```python
from build123d import *

# Parameters (mm, degrees)
F0_R     = 31.5
F0_R_2   = 26.5
F1_DEPTH = 25
F2_R     = 37
F2_R_2   = 31.5
F2_R_3   = 26.5
F3_DEPTH = 5
F4_R     = 1
F5_R     = 1
F6_R     = 5


with BuildPart() as f1:
    # F0 (on Top) → F1 (new body)
    with BuildSketch(Plane.XY):
        Circle(F0_R)
        Circle(F0_R_2, mode=Mode.SUBTRACT)
    extrude(amount=F1_DEPTH)

    # F2 (on face) → F3 (join)
    with BuildSketch(Plane.XY.offset(25)):
        Circle(F2_R)
        Circle(F2_R_2, mode=Mode.SUBTRACT)
        Circle(F2_R_2)
        Circle(F2_R_3, mode=Mode.SUBTRACT)
        Circle(F2_R_3)
    extrude(amount=F3_DEPTH)

    # F4
    f4_edges = [f1.edges().sort_by_distance(p)[0] for p in [
        (-37, 0, 30),
    ]]
    fillet(f4_edges, radius=F4_R)

    # F5
    f5_edges = [f1.edges().sort_by_distance(p)[0] for p in [
        (-31.5, 0, 0),
    ]]
    fillet(f5_edges, radius=F5_R)

    # F6
    f6_edges = [f1.edges().sort_by_distance(p)[0] for p in [
        (-26.5, 0, 25),
    ]]
    fillet(f6_edges, radius=F6_R)


solid = f1.part
```
Geometry check sheet. Reference: the model listing, model coordinates, mm. A direction names the side the tool comes from. Round coordinates to 2 decimals unless told otherwise and drop trailing zeros. Order: outer loops, then holes, each group sorted by start corner. A loop starts at its lowest first (then second) coordinate and runs counter-clockwise, first axis right, second up. Notation, with made-up numbers: M -12,44.25 L 5,44.25 A25 cw 5,79.25 Z; hole C 56,-24 d1. An arc over 180 degrees is marked long. Answer as CSV lines item,"result".
1) Tool access check on faces 1 (the face through (-8.02, -36.12, 26.97)), 2 (the face through (27, 17, 25)). Record the directions out of +Z, -Z, +X, -X, +Y, -Y that give a thin tool (end or side, any length) a straight path to the whole face; none if there is none.
Entries:
face 1,"+Z, -Z"
face 2,"-Z"
2) Sectioned sample at A-A on x = 0. Record the cut outline in (y, z).
Entries:
outline,"M -37,25 L -31.5,25 L -31.5,1 A1 ccw -30.5,0 L -26.5,0 L -26.5,20 A5 cw -21.5,25 L 21.5,25 A5 cw 26.5,20 L 26.5,0 L 30.5,0 A1 ccw 31.5,1 L 31.5,25 L 37,25 L 37,29 A1 ccw 36,30 L -36,30 A1 ccw -37,29 Z"
3) Sectioned sample at D-D on z = 26. Record the cut outline in (x, y), and give its area (3 significant figures).
Entries:
outline,"C 0,0 d74"
area,"4,300 mm2"
4) Mould release check, pull along Y, two halves, no side actions. Record for faces 3 (the face through (14.246, 22.345, 9.86)), 4 (the face through (-4.101, 31.232, 12.832)), 5 (the face through (-23, 14, 0)): +Y half, -Y half, draft (parallel to the pull), parting line (faces both ways), or undercut.
Entries:
face 3,"undercut"
face 4,"parting line"
face 5,"draft"
5) Sectioned sample at C-C on z = 10.5. Record the cut outline in (x, y), and give its area (3 significant figures).
Entries:
outline,"C 0,0 d63; hole C 0,0 d53"
area,"911 mm2"
6) Thickness scan on probe 1 along Y at (x, z) = (0, 10.25); probe 2 along X at (y, z) = (4, 19.5) (3 decimals); probe 3 along Z at (x, y) = (14.5, 1.5). Record the ranges inside material, lowest first. Write a range as [from, to].
Entries:
probe 1,"[-31.5, -26.5], [26.5, 31.5]"
probe 2,"[-31.245, -26.196], [26.196, 31.245]"
probe 3,"[25, 30]"
7) Gauge pin test, flat ends, axial feed: pin 1 Ø5 at (x, y) = (23, 4.5) entering from -Z; pin 2 Ø4 at (y, z) = (-11.5, 11) entering from +X; pin 3 Ø3 at (x, z) = (-10, 21.5) entering from +Y. Record the tip position at first contact, or that the pin passes through.
Entries:
pin 1,"z = 22.31"
pin 2,"x = 30.03"
pin 3,"y = 30.33"
